The listing builds one solid part. Answer for the finished solid, in the listing's coordinates (mm). A direction names the side the tool comes from. Give positions to 0.01 mm unless a question says otherwise; leave off trailing zeros. Loops run counter-clockwise (first coordinate to the right, second up) from the corner with the lowest first, then second, coordinate; pieces in that order, holes last.
Item 1: A tool of negligible diameter and unlimited length cuts with its end or side. For faces 1 (the face through (20.638, 17, 6)), 2 (the face through (28.575, 5, 6)), 3 (the face through (29.425, 11.797, 12.575)), from which of +Z, -Z, +X, -X, +Y, -Y can it reach the whole face along a straight path? Write none if from no direction.
Item 2: The mould has two halves that part along Z. Classify faces 4 (the face through (29.425, 11.797, 0.125)), 5 (the face through (7.508, 6.266, 9.624)), 6 (the face through (34, 12.7, 6)), 7 (the face through (19.788, 13.603, 12.575)): pulls with the +Z half, pulls with the -Z half, needs draft (parallel to the pull), parting line crosses it, or undercut.
Item 3: Each of these flat-tipped pins is pushed along its axis until it touches: pin 1 Ø4 at (y, z) = (6, 7.5) entering from +X (3 decimals); pin 2 Ø5 at (x, z) = (35.5, 6) entering from -Y; pin 3 Ø1.1 at (y, z) = (16.5, 7) entering from -X. Where does it stop, or does it pass through?
Item 4: Consider line 1 along X through (y, z) = (3.25, 6.5) (3 decimals); line 2 along Y through (x, z) = (15, 7); line 3 along X through (y, z) = (6.5, 0.5) (3 decimals). Determine where each line is inside the solid, lowest interval first.
Item 5: Section D-D, the plane y = 17.5 is taken. Give the vertices of the cut face in (x, z).
from build123d import *

# Parameters (mm, degrees)
F1_DEPTH = 12.7
F2_R     = 0.762
F3_R     = 3.302
F4_DEPTH = 19.051
F5_SIZE  = 0.381
F6_SIZE  = 0.254


with BuildPart() as f1:
    # F0 (on Top) → F1 (new body)
    with BuildSketch(Plane.XY):
        with BuildLine():
            Line((0, 12.7), (0, 0))
            Line((0, 0), (28.575, 0))
            Line((28.575, 0), (28.575, 9.398))
            ThreePointArc((28.575, 9.398), (29.542133, 11.732867), (31.877, 12.7))
            Line((31.877, 12.7), (36.5125, 12.7))
            Line((36.5125, 12.7), (36.5125, 19.05))
            Line((36.5125, 19.05), (20.6375, 19.05))
            Line((20.6375, 19.05), (20.6375, 16.002))
            ThreePointArc((20.6375, 16.002), (19.670367, 13.667133), (17.3355, 12.7))
            Line((17.3355, 12.7), (0, 12.7))
        make_face()
    extrude(amount=F1_DEPTH)

    # F2
    f2_edges = [f1.edges().sort_by_distance(p)[0] for p in [
        (28.575, 0, 6.35),
        (0, 0, 6.35),
        (0, 12.7, 6.35),
        (20.6375, 19.05, 6.35),
        (36.5125, 19.05, 6.35),
    ]]
    fillet(f2_edges, radius=F2_R)

    # F3 (on face) → F4 (cut, through all)
    with BuildSketch(Plane.XZ):
        with Locations((7.9375, 6.35)):
            Circle(F3_R)
    extrude(amount=-F4_DEPTH, mode=Mode.SUBTRACT)

    # F5
    f5_edges = [f1.edges().sort_by_distance(p)[0] for p in [
        (4.6355, 12.7, 6.35),
        (4.6355, 0, 6.35),
    ]]
    chamfer(f5_edges, length=F5_SIZE)

    # F6
    f6_edges = [f1.edges().sort_by_distance(p)[0] for p in [
        (9.04875, 12.7, 12.7),
        (0.223185, 12.476815, 12.7),
        (19.670367, 13.667133, 12.7),
        (0, 6.35, 12.7),
        (20.6375, 17.145, 12.7),
        (0.223185, 0.223185, 12.7),
        (20.860685, 18.826815, 12.7),
        (14.2875, 0, 12.7),
        (28.575, 19.05, 12.7),
        (28.351815, 0.223185, 12.7),
        (36.289315, 18.826815, 12.7),
        (28.575, 5.08, 12.7),
        (36.5125, 15.494, 12.7),
        (29.542133, 11.732867, 12.7),
        (34.19475, 12.7, 12.7),
        (9.04875, 12.7, 0),
        (0.223185, 12.476815, 0),
        (19.670367, 13.667133, 0),
        (0, 6.35, 0),
        (20.6375, 17.145, 0),
        (0.223185, 0.223185, 0),
        (20.860685, 18.826815, 0),
        (14.2875, 0, 0),
        (28.575, 19.05, 0),
        (28.351815, 0.223185, 0),
        (36.289315, 18.826815, 0),
        (28.575, 5.08, 0),
        (36.5125, 15.494, 0),
        (29.542133, 11.732867, 0),
        (34.19475, 12.7, 0),
    ]]
    chamfer(f6_edges, length=F6_SIZE)


solid = f1.part
Worked answers:
1. face 1: +Z, -Z, -X, +Y
1. face 2: +Z, -Z, +X, -Y
1. face 3: +Z, +X, -Y
2. face 4: pulls with the -Z half
2. face 5: undercut
2. face 6: needs draft
2. face 7: pulls with the +Z half
3. pin 1: stops at x = 28.575
3. pin 2: stops at y = 12.7
3. pin 3: stops at x = 20.64
4. line 1: x = 0 to 4.639, 11.236 to 28.575
4. line 2: y = 0 to 12.7
4. line 3: x = 0 to 28.575
5. outline: (20.64, 0.25) - (20.89, 0) - (36.26, 0) - (36.51, 0.25) - (36.51, 12.45) - (36.26, 12.7) - (20.89, 12.7) - (20.64, 12.45) - close
